from build123d import *

# Parameters (mm, degrees)
F0_R      = 7.2
F0_R_2    = 4.75
F0_R_3    = 4.5
F1_DEPTH  = 6
F1_FACE_R = 4.5
F2_DEPTH  = 6.001
F3_SIZE2  = 0.5
F3_SIZE   = 0.5


with BuildPart() as f1:
    # F0 (on Front) → F1 (new body)
    with BuildSketch(Plane.XZ):
        with Locations((-0.020111, 0.117168)):
            Circle(F0_R)
        Circle(F0_R_2, mode=Mode.SUBTRACT)
        Circle(F0_R_3)
    extrude(amount=F1_DEPTH)

    # F1_face (on face) → F2 (cut, through all)
    with BuildSketch(Plane.XZ.offset(6)):
        Circle(F1_FACE_R)
    extrude(amount=-F2_DEPTH, mode=Mode.SUBTRACT)

    # F3
    f3_edges = [f1.edges().sort_by_distance(p)[0] for p in [
        (4.75, -3, 0),
        (-4.75, 0, 0),
        (-4.75, -6, 0),
    ]]
    chamfer(f3_edges, length=F3_SIZE, length2=F3_SIZE2)


solid = f1.part
Can you work these out from the model? Positions are in its coordinate system, mm. Give positions to 0.01 mm unless a question says otherwise; leave off trailing zeros. Loops run counter-clockwise (first coordinate to the right, second up) from the corner with the lowest first, then second, coordinate; pieces in that order, holes last. Notation, with made-up numbers: M 74,-12 L 123,-12 A14 ccw 123,-7 Z; hole C 18.5,-34.5 d4. An arc over 180 degrees is marked long. One line per item, written item: value. Start each with the question number.
1) If we section it at A-A, the plane x = 0: Write out the boundary of the cut face in (y, z), and give its area (3 significant figures).
2) I'm going to push flat-ended pins straight in: pin 1 (2 mm diameter, centred on x = -4.5, y = -2, fed in from +Z); pin 2 (1.5 mm diameter, centred on y = -1, z = -3, fed in from -X). Where does each tip first touch, or does it pass through?
3) Thinking about a two-plate mould opening in Z: for faces 1 (the face through (2.192, -2.965, -4.214)), 2 (the face through (2.1, -6, 5)), 3 (the face through (-1.58, -2.96, -6.91)), which applies, +Z half, -Z half, draft (parallel to the pull), parting line (faces both ways), or undercut?
4) If I drill on line 1 (Z direction, x = 0, y = -3.2); line 2 (X direction, y = -1.85, z = -3.5); line 3 (Z direction, x = -1, y = -2.5), over which ranges is the centre line in solid material (lowest first)? Write a range as [from, to].
5) If we section it at B-B, the plane y = -4.7: Write out the boundary of the cut face in (x, z).
6) If we section it at C-C, the plane z = 5.5: Write out the boundary of the cut face in (x, y), and give its area (3 significant figures).
Completed:
1. outline: M -6,-7.08 L 0,-7.08 L 0,-5.25 L -0.5,-4.75 L -5.5,-4.75 L -6,-5.25 Z; M -6,5.25 L -5.5,4.75 L -0.5,4.75 L 0,5.25 L 0,7.32 L -6,7.32 Z
1. area: 28.9 mm^2
2. pin 1: stops at z = 6.42
2. pin 2: stops at x = -6.82
3. face 1: undercut
3. face 2: draft
3. face 3: parting line
4. line 1: z = [-7.08, -4.75], [4.75, 7.32]
4. line 2: x = [-6.25, -3.21], [3.21, 6.21]
4. line 3: z = [-7.02, -4.64], [4.64, 7.25]
5. outline: C -0.02,0.12 d14.4; hole C 0,0 d9.5
6. outline: M -4.8,-6 L 4.76,-6 L 4.76,0 L -4.8,0 Z
6. area: 57.4 mm^2
